Read the model definition and answer for the solid it produces. Units are mm, in the model's axes. A direction names the side the tool comes from. Give positions to 0.01 mm unless a question says otherwise; leave off trailing zeros. Order: outer loops, then holes, each group sorted by start corner. A loop starts at its lowest first (then second) coordinate and runs counter-clockwise, first axis right, second up.
Item 1: Given pin 1 Ø3 at (x, y) = (7, -11.5) entering from +Z; pin 2 Ø3.5 at (x, y) = (2, -2) entering from -Z; pin 3 Ø6 at (x, z) = (6, -4) entering from -Y; pin 4 Ø5 at (x, z) = (-1, 0) entering from -Y, each flat-ended and moving along its own axis, determine where each tip first touches the part or whether it passes through.
Item 2: A cutting plane is placed at B-B (z = 4.5). Write down the section's boundary in (x, y) (1 decimal).
Item 3: The mould has two halves that part along X. Classify faces 4 (the face through (-5.08, -16, 0)), 5 (the face through (1, -14.22, 0)), 6 (the face through (-2.3, 2.29, -0.1)): +X half, -X half, draft (parallel to the pull), parting line (faces both ways), or undercut.
Item 4: Find the intervals of material crossed by line 1 along X through (y, z) = (-2, -2) (3 decimals); line 2 along Y through (x, z) = (4.5, -5.5); line 3 along Y through (x, z) = (1.5, 0.25), in increasing order.
Item 5: A cutting plane is placed at C-C (y = 6.5). Write down the section's boundary in (x, z) (3 decimals), plus the area to 3 significant figures.
Item 6: Which of the six approach directions +Z, -Z, +X, -X, +Y, -Y give full straight-line access (tool end or side, diameter ignored) to faces 1 (the face through (0, -4, 6.35)), 2 (the face through (-3.168, 8.169, -0.08)), 3 (the face through (0.38, -16, 0))?
Item 7: A cutting plane is placed at A-A (x = 1). Write down the section's boundary in (y, z), plus the area to 3 significant figures.
Item 8: A cutting plane is placed at D-D (x = -1). Write down the section's boundary in (y, z) (3 decimals).
from build123d import *

# Parameters (mm, degrees)
SKETCH1_W                = 19.43
SKETCH1_H                = 15.62
BOSS_EXTRUDE1_DEPTH      = 2.29
SKETCH5_W                = 15.25
SKETCH5_H                = 12.7
BOSS_EXTRUDE2_DEPTH      = 7.11
SKETCH6_W                = 12.7
SKETCH6_H                = 6
BOSS_EXTRUDE3_DEPTH      = 7.11
SKETCH7_W                = 0.76
SKETCH7_H                = 2.03
BOSS_EXTRUDE4_DEPTH      = 3.94
BOSS_EXTRUDE5_DEPTH      = 5.715
BOSS_EXTRUDE5_DEPTH_BACK = 5.715


with BuildPart() as part:
    # Sketch1 → Boss-Extrude1 (new body)
    with BuildSketch(Plane(origin=(0, 0, 0), x_dir=(1, 0, 0), z_dir=(0, 1, 0))):
        Rectangle(SKETCH1_W, SKETCH1_H)
    extrude(amount=BOSS_EXTRUDE1_DEPTH)

    # Sketch5 → Boss-Extrude2 (add)
    with BuildSketch(Plane.XZ):
        Rectangle(SKETCH5_W, SKETCH5_H)
    extrude(amount=BOSS_EXTRUDE2_DEPTH)

    # Sketch6 → Boss-Extrude3 (add)
    with BuildSketch(Plane.XZ.offset(7.11)):
        Rectangle(SKETCH6_W, SKETCH6_H)
    extrude(amount=BOSS_EXTRUDE3_DEPTH)

    # Sketch7 → Boss-Extrude4 (add)
    with BuildSketch(Plane.XZ.offset(14.22)):
        Rectangle(SKETCH7_W, SKETCH7_H)
        with Locations((-4.7, 0)):
            Rectangle(SKETCH7_W, SKETCH7_H)
        with Locations((4.7, 0)):
            Rectangle(SKETCH7_W, SKETCH7_H)
    extrude(amount=BOSS_EXTRUDE4_DEPTH)

    # Sketch8 → Boss-Extrude5 (add, two sides: drawn at the far end of the back side and taken through both)
    with BuildSketch(Plane.XY.offset(-BOSS_EXTRUDE5_DEPTH_BACK)):
        Polygon((-1.162073149, -3.20490485), (1.162073149, -2.79509515), (-1.851354952, 14.29490485), (-4.175501249, 13.88509515), align=None)
    extrude(amount=BOSS_EXTRUDE5_DEPTH + BOSS_EXTRUDE5_DEPTH_BACK)


solid = part.part
Response values:
1. pin 1: stops at z = 3
1. pin 2: stops at z = -6.35
1. pin 3: stops at y = -14.22
1. pin 4: stops at y = -18.16
2. outline: (-9.7, 0) - (-7.6, 0) - (-7.6, -7.1) - (7.6, -7.1) - (7.6, 0) - (9.7, 0) - (9.7, 2.3) - (0.3, 2.3) - (-1.9, 14.3) - (-4.2, 13.9) - (-2.1, 2.3) - (-9.7, 2.3) - close
3. face 4: -X half
3. face 5: undercut
3. face 6: draft
4. line 1: x = -7.625 to 7.625
4. line 2: y = -7.11 to 2.29
4. line 3: y = -14.22 to 2.29
5. outline: (-2.873, -5.715) - (-0.477, -5.715) - (-0.477, 5.715) - (-2.873, 5.715) - close
5. area: 27.4 mm2
6. face 1: +Z, +X, -X, -Y
6. face 2: +Z, -Z, -X
6. face 3: +Z, -Z, -Y
7. outline: (-14.22, -3) - (-7.11, -3) - (-7.11, -6.35) - (0, -6.35) - (0, -7.81) - (2.29, -7.81) - (2.29, 7.81) - (0, 7.81) - (0, 6.35) - (-7.11, 6.35) - (-7.11, 3) - (-14.22, 3) - close
7. area: 169 mm2
8. outline: (-14.22, -3) - (-7.11, -3) - (-7.11, -6.35) - (0, -6.35) - (0, -7.81) - (2.29, -7.81) - (2.29, -5.715) - (9.467, -5.715) - (9.467, 5.715) - (2.29, 5.715) - (2.29, 7.81) - (0, 7.81) - (0, 6.35) - (-7.11, 6.35) - (-7.11, 3) - (-14.22, 3) - close
